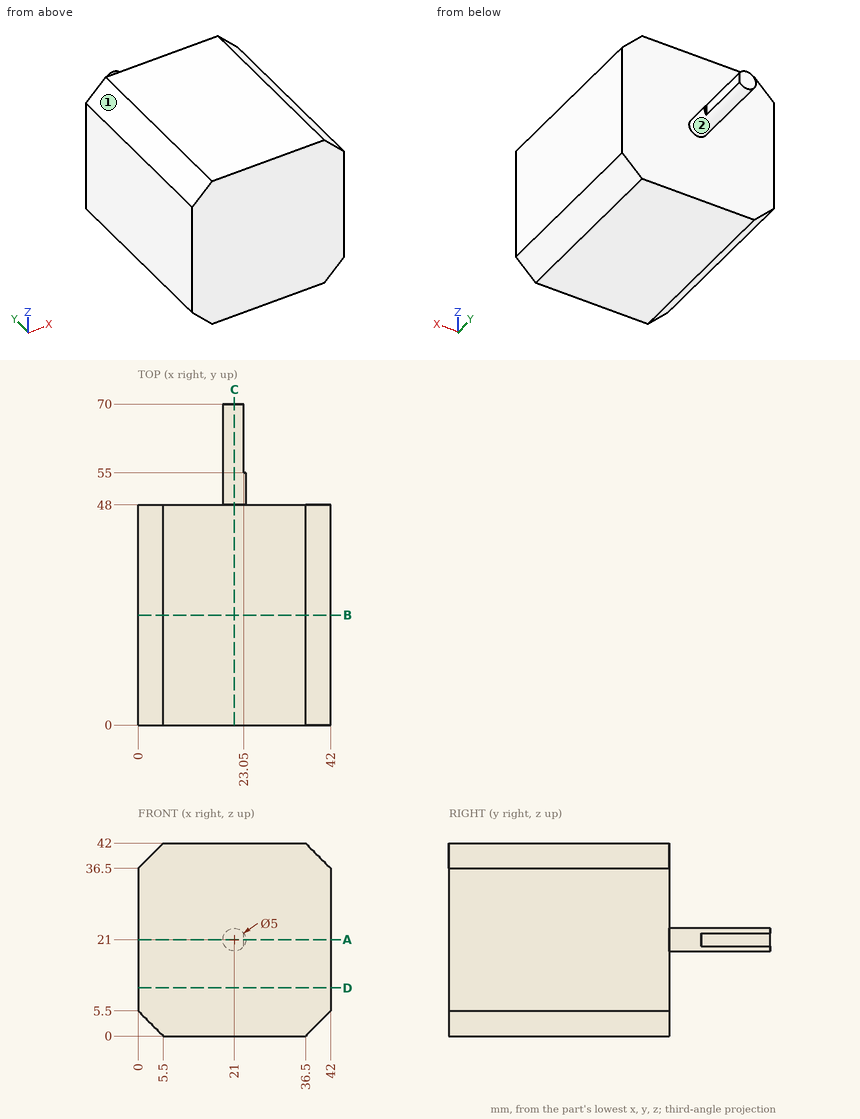
Could you check a few things on this drawing? It's one solid part, dimensions in mm from its lowest x, y, z. A direction names the side the tool comes from. Round coordinates to 2 decimals unless told otherwise and drop trailing zeros. Order: outer loops, then holes, each group sorted by start corner. A loop starts at its lowest first (then second) coordinate and runs counter-clockwise, first axis right, second up. Notation, with made-up numbers: M 71.5,25.5 L 112.5,25.5 A17 ccw 112.5,53.5 Z; hole C 28,3.5 d11. An arc over 180 degrees is marked long. One line per question, with ' | ' between items. Start each with the question number.
(1) Please list where these lines run through material, in increasing order: line 1 along Y through (x, z) = (37, 23); line 2 along X through (y, z) = (40, 4.5); line 3 along X through (y, z) = (39.5, 37).
(2) Suppose I cut it at C-C on x = 21. List the corners of the cut face in (y, z) for me.
(3) Suppose I cut it at A-A on z = 21. List the corners of the cut face in (x, y) for me, then the cut area to 3 significant figures.
(4) Suppose I cut it at D-D on z = 10.5. List the corners of the cut face in (x, y) for me, then the cut area to 3 significant figures.
(5) Suppose I cut it at B-B on y = 24. List the corners of the cut face in (x, z) for me, then the cut area to 3 significant figures.
(6) For P1, Ø2, axis at x = 13, z = 19, coming from the +Y side; P2, Ø2.5, axis at y = 63, z = 21, coming from the +X side, each with a flat end and sliding along its axis, tell me the tip position at first contact or that it passes through.
(7) For the marked faces 1 and 2, which set-ups out of +Z, -Z, +X, -X, +Y, -Y let a thin tool reach every point of the face, with its end or its side?
Geometry results:
1) line 1: 0 to 48 | line 2: 1 to 41 | line 3: 0.5 to 41.5
2) outline: M 0,0 L 48,0 L 48,18.5 L 70,18.5 L 70,23.5 L 48,23.5 L 48,42 L 0,42 Z
3) outline: M 0,0 L 42,0 L 42,48 L 23.5,48 L 23.5,55 L 23.05,55 L 23.05,70 L 18.5,70 L 18.5,48 L 0,48 Z | area: 2,120 mm²
4) outline: M 0,0 L 42,0 L 42,48 L 0,48 Z | area: 2,020 mm²
5) outline: M 0,5.5 L 5.5,0 L 36.5,0 L 42,5.5 L 42,36.5 L 36.5,42 L 5.5,42 L 0,36.5 Z | area: 1,700 mm²
6) P1: y = 48 | P2: x = 23.05
7) face 1: +Z, -X, +Y, -Y | face 2: +Y
